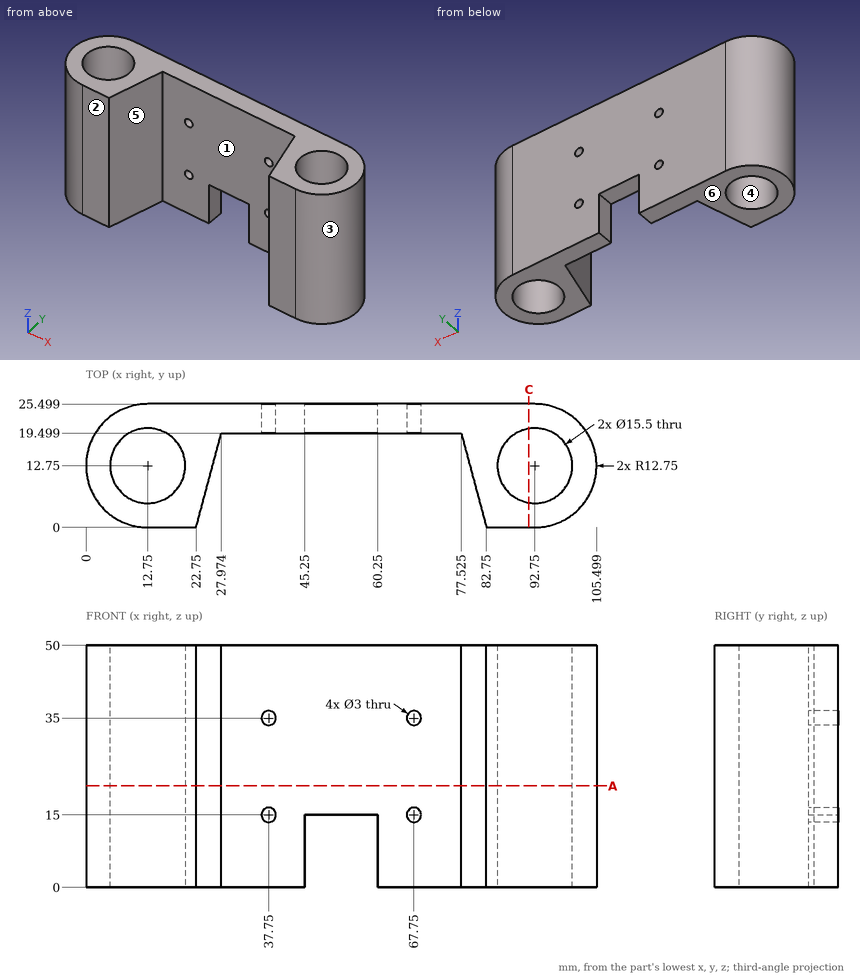
Here's the drawing with two shaded views (mm, measured from the low corner). I have some questions. A direction names the side the tool comes from. Round coordinates to 2 decimals unless told otherwise and drop trailing zeros. Loops run counter-clockwise (first coordinate to the right, second up) from the corner with the lowest first, then second, coordinate; pieces in that order, holes last.
Item 1: Please list where these lines run through material, in increasing order: L1, parallel to Y at x = 92.5, z = 24.5 (1 decimal); L2, parallel to X at y = 11.5, z = 15; L3, parallel to X at y = 8, z = 33.5 (1 decimal).
Item 2: Suppose I cut it at A-A, the plane z = 21. State how many separate pieces and enclosed holes the cut face has, then the cut area to 4 significant figures.
Item 3: Will these pins go through, and if not, where does the flat tip stop? pin 1 Ø2.5 at (x, z) = (37.75, 15) entering from +Y; pin 2 Ø3 at (y, z) = (21.5, 7.5) entering from -X; pin 3 Ø12 at (x, z) = (61.5, 34.5) entering from -Y; pin 4 Ø1.8 at (y, z) = (22, 5.5) entering from +X (1 decimal).
Item 4: Suppose I cut it at C-C, the plane x = 91.5. Write out the boundary of the cut face in (y, z).
Item 5: Which directions (+Z, -Z, +X, -X, +Y, -Y) give clear straight access to the entire face, cutting with the end or side of a thin tool? Please do the marked faces 1 and 2.
Item 6: If we mould it in two halves opening along X, with no side actions, what happens to the marked faces 3, 4, 5 and 6? For each: +X half, -X half, draft (parallel to the pull), parting line (faces both ways), or undercut.
Reported:
1. L1: y = 0 to 5, 20.5 to 25.5
1. L2: x = 0.06 to 5.1, 20.4 to 25.83, 79.67 to 85.1, 100.4 to 105.44
1. L3: x = 0.9 to 6.6, 18.9 to 24.9, 80.6 to 86.6, 98.9 to 104.6
2. separate pieces: 1
2. enclosed holes: 2
2. area: 1,105 mm2
3. pin 1: passes through
3. pin 2: stops at x = 2.26
3. pin 3: stops at y = 19.5
3. pin 4: stops at x = 102.4
4. outline: (0, 0) - (5.1, 0) - (5.1, 50) - (0, 50) - close; (20.4, 0) - (25.5, 0) - (25.5, 50) - (20.4, 50) - close
5. face 1: +Z, -Z, -Y
5. face 2: +Z, -Z, +X, -X, -Y
6. face 3: +X half
6. face 4: undercut
6. face 5: undercut
6. face 6: draft
